Geometry check sheet. Reference: the model listing, model coordinates, mm. Give positions to 0.01 mm unless a question says otherwise; leave off trailing zeros. Write each loop counter-clockwise with the first axis right and the second up, starting at its lowest first coordinate (ties: lowest second). Pieces come first, ordered by that corner, then holes. Notation, with made-up numbers: M -8,77 L 13,77 A18 ccw 13,90 Z; hole C 67.5,51 d11. An arc over 180 degrees is marked long. Write each question's results on one line, items separated by ' | '.
```python
from build123d import *

# Parameters (mm, degrees)
SKETCH1_W           = 120
SKETCH1_H           = 195
BOSS_EXTRUDE1_DEPTH = 10
SKETCH2_R           = 2.75
CUT_EXTRUDE1_DEPTH  = 11
SKETCH3_R           = 4.6
CUT_EXTRUDE2_DEPTH  = 5


with BuildPart() as part:
    # Sketch1 → Boss-Extrude1 (new body)
    with BuildSketch(Plane(origin=(0, 0, 0), x_dir=(1, 0, 0), z_dir=(0, 1, 0))):
        with Locations((-17.427799272, -26.251292201)):
            Rectangle(SKETCH1_W, SKETCH1_H)
    extrude(amount=BOSS_EXTRUDE1_DEPTH)

    # Sketch2 → Cut-Extrude1 (cut, through all)
    with BuildSketch(Plane(origin=(0, 10, 0), x_dir=(-1, 0, 0), z_dir=(0, 1, 0))):
        with Locations((-22.572200728, 118.751292201)):
            Circle(SKETCH2_R)
        with Locations((57.427799272, 118.751292201)):
            Circle(SKETCH2_R)
        with Locations((-22.572200728, 3.751292201)):
            Circle(SKETCH2_R)
        with Locations((57.427799272, 3.751292201)):
            Circle(SKETCH2_R)
        with Locations((-22.572200728, -66.248707799)):
            Circle(SKETCH2_R)
        with Locations((57.427799272, -66.248707799)):
            Circle(SKETCH2_R)
    extrude(amount=-CUT_EXTRUDE1_DEPTH, mode=Mode.SUBTRACT)

    # Sketch3 → Cut-Extrude2 (cut)
    with BuildSketch(Plane(origin=(0, 10, 0), x_dir=(1, 0, 0), z_dir=(0, 1, 0))):
        with Locations((22.572200728, -3.751292201)):
            Circle(SKETCH3_R)
        with Locations((-57.427799272, -3.751292201)):
            Circle(SKETCH3_R)
        with BuildLine():
            Line((-62.027799272, 66.248707799), (-62.027799272, 71.248707799))
            Line((-62.027799272, 71.248707799), (-52.827799272, 71.248707799))
            Line((-52.827799272, 71.248707799), (-52.827799272, 66.248707799))
            ThreePointArc((-52.827799272, 66.248707799), (-57.427799272, 61.648707799), (-62.027799272, 66.248707799))
        make_face()
        with BuildLine():
            Line((17.972200728, 66.248707799), (17.972200728, 71.248707799))
            Line((17.972200728, 71.248707799), (27.172200728, 71.248707799))
            Line((27.172200728, 71.248707799), (27.172200728, 66.248707799))
            ThreePointArc((27.172200728, 66.248707799), (22.572200728, 61.648707799), (17.972200728, 66.248707799))
        make_face()
        with BuildLine():
            Line((-62.027799272, -118.751292201), (-62.027799272, -123.751292201))
            Line((-62.027799272, -123.751292201), (-52.827799272, -123.751292201))
            Line((-52.827799272, -123.751292201), (-52.827799272, -118.751292201))
            ThreePointArc((-52.827799272, -118.751292201), (-57.427799272, -114.151292201), (-62.027799272, -118.751292201))
        make_face()
        with BuildLine():
            Line((17.972200728, -118.751292201), (17.972200728, -123.751292201))
            Line((17.972200728, -123.751292201), (27.172200728, -123.751292201))
            Line((27.172200728, -123.751292201), (27.172200728, -118.751292201))
            ThreePointArc((27.172200728, -118.751292201), (22.572200728, -114.151292201), (17.972200728, -118.751292201))
        make_face()
    extrude(amount=-CUT_EXTRUDE2_DEPTH, mode=Mode.SUBTRACT)


solid = part.part
```
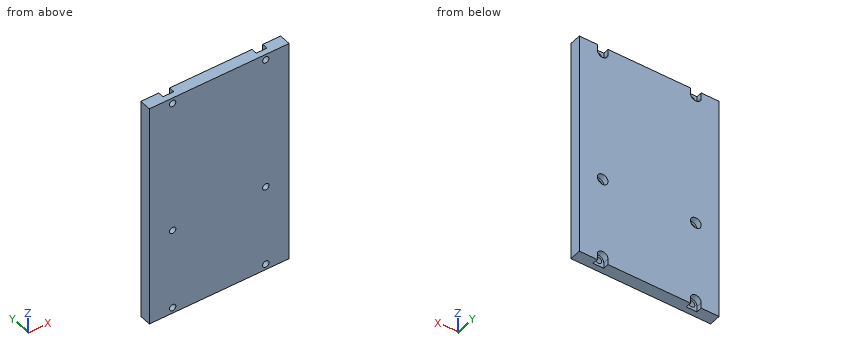
Q1. Depth check by flat-ended pin: P1, Ø8.5, axis at x = -57.43, z = 3.75, coming from the +Y side. Enter the tip coordinate at first touch or a pass-through.
Answer key:
P1: stops at y = 5
Q2. Material ranges on probe 1 along X at (y, z) = (8, 115); probe 2 along Z at (x, y) = (25, 3.5); probe 3 along X at (y, z) = (5.25, 1), recorded low to high. Write a range as [from, to].
Answer key:
probe 1: x = [-77.43, -60.09], [-54.77, 19.91], [25.23, 42.57] | probe 2: z = [-71.25, -67.54], [-64.96, 2.46], [5.04, 117.46], [120.04, 123.75] | probe 3: x = [-77.43, -61.11], [-53.74, 18.89], [26.26, 42.57]
Q3. Section check A-A (y = 6.75). Enter the section's corners in (x, z), then the cut area to 3 significant figures.
Answer key:
outline: M -77.43,-71.25 L -62.03,-71.25 L -62.03,-66.25 A4.6 cw -52.83,-66.25 L -52.83,-71.25 L 17.97,-71.25 L 17.97,-66.25 A4.6 cw 27.17,-66.25 L 27.17,-71.25 L 42.57,-71.25 L 42.57,123.75 L 27.17,123.75 L 27.17,118.75 A4.6 cw 17.97,118.75 L 17.97,123.75 L -52.83,123.75 L -52.83,118.75 A4.6 cw -62.03,118.75 L -62.03,123.75 L -77.43,123.75 Z; hole C -57.43,3.75 d9.2; hole C 22.57,3.75 d9.2 | area: 23,000 mm2
